Job drawing, mm, ordinate dimensions from the low corner. One solid piece. Round coordinates to 2 decimals unless told otherwise and drop trailing zeros. Loops run counter-clockwise (first coordinate to the right, second up) from the corner with the lowest first, then second, coordinate; pieces in that order, holes last.
1) Probe line 1 (Y direction, x = 11, z = 22); line 2 (Y direction, x = 23.5, z = 58.5); line 3 (X direction, y = 20, z = 14). List the from-to ranges inside material, lowest first.
2) Band-saw the part on B-B, the plane y = 3.5. Write the cut outline in (x, z).
3) Band-saw the part on C-C, the plane x = 92.5. Write the cut outline in (y, z).
4) Drop flat-ended pins along their axis: P1, Ø1, axis at x = 35, z = 40.5, coming from the -Y side; P2, Ø3, axis at y = 17.5, z = 12, coming from the -X side; P3, Ø1.5, axis at y = 13, z = 43.5, coming from the +X side; P4, Ø2, axis at y = 4.5, z = 32.5, coming from the -X side. Give the stop position or say it passes through.
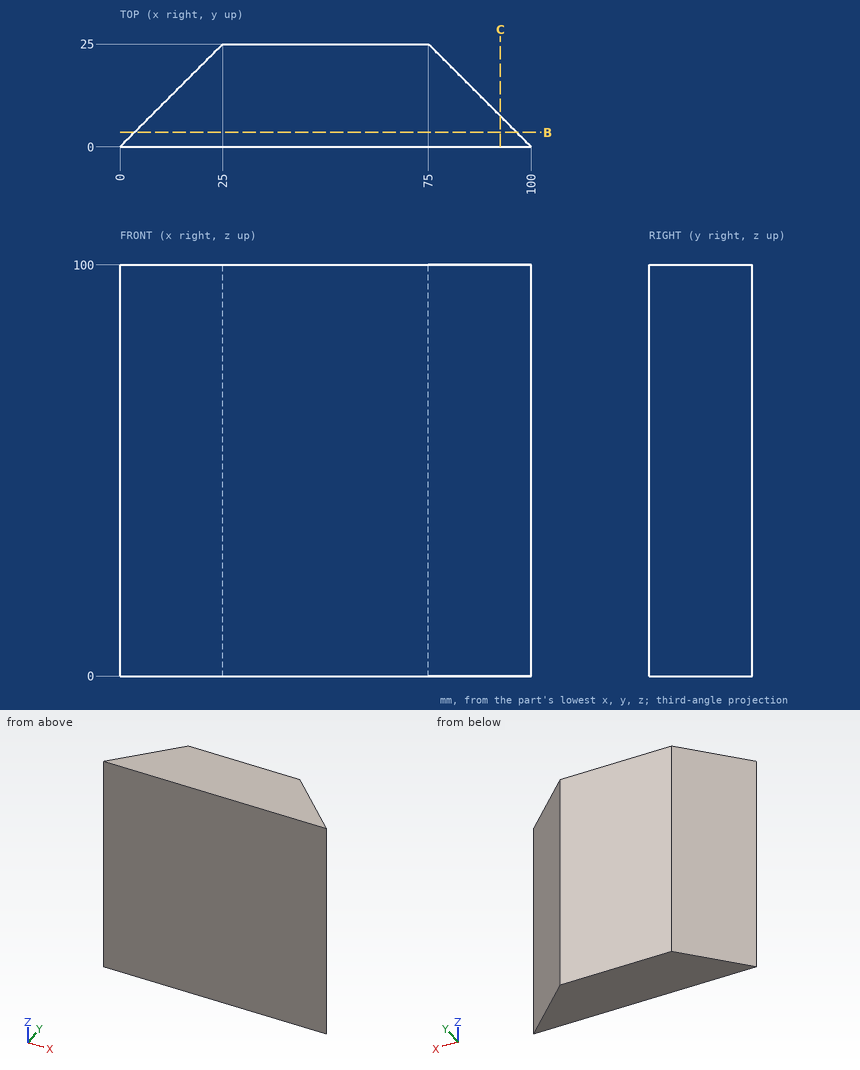
Reported:
1. line 1: y = 0 to 11
1. line 2: y = 0 to 23.5
1. line 3: x = 20 to 80
2. outline: (3.5, 0) - (96.5, 0) - (96.5, 100) - (3.5, 100) - close
3. outline: (0, 0) - (7.5, 0) - (7.5, 100) - (0, 100) - close
4. P1: stops at y = 0
4. P2: stops at x = 16
4. P3: stops at x = 87.75
4. P4: stops at x = 3.5
